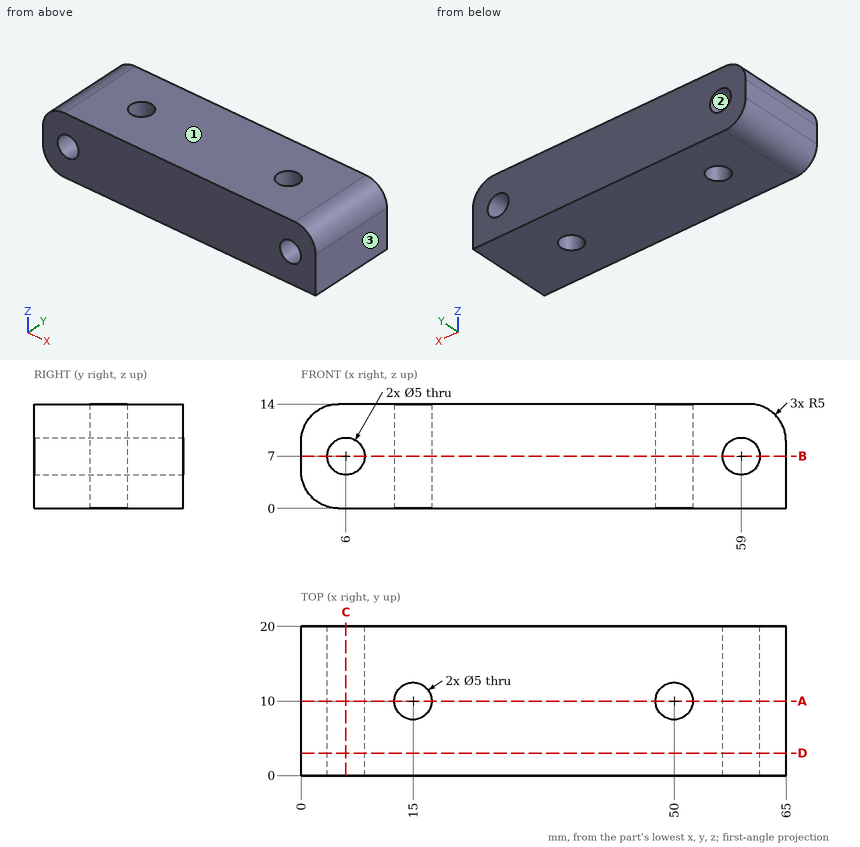
Input: dimensioned drawing with shaded views. Units: mm. Origin: part minimum x, y, z. Round coordinates to 2 decimals unless told otherwise and drop trailing zeros. Order: outer loops, then holes, each group sorted by start corner. A loop starts at its lowest first (then second) coordinate and runs counter-clockwise, first axis right, second up. Notation, with made-up numbers: (-2.75, 45) - (45.25, 45) arc R24 ccw to (45.25, 79) - close; hole circle Ø2 at (56, -39). An arc over 180 degrees is marked (long way). Answer as a JSON object with one key per item and string values. Group by question number.
(1) Cut plane C-C (x = 6). Return loops of the section in (y, z).
(2) Cut plane A-A (y = 10). Return loops of the section in (x, z).
(3) Pin query (flat end, axial travel): P1, Ø2, axis at y = 3, z = 2.5, coming from the -X side; P2, Ø1, axis at y = 3.5, z = 1.5, coming from the -X side. Return the tip coordinate at first contact, or that it passes through.
(4) Cut plane D-D (y = 3). Return loops of the section in (x, z), then the cut area to 3 significant figures.
(5) Cut plane B-B (z = 7). Return loops of the section in (x, y).
(6) Material intervals for probe 1 along Z at (x, y) = (59, 4); probe 2 along Y at (x, z) = (50, 8); probe 3 along X at (y, z) = (6.75, 5.25), sorted ascending. Write a range as from..to.
(7) Draft query along X for the marked faces 1, 2 and 3. Return one class per face: released by +X, released by -X, zero draft, split by the parting line, or undercut.
Here are the results:
{
 "1": {"outline": "(0, 0) - (20, 0) - (20, 4.5) - (0, 4.5) - close; (0, 9.5) - (20, 9.5) - (20, 14) - (0, 14) - close"},
 "2": {"outline": "(0, 5) arc R5 ccw to (5, 0) - (12.5, 0) - (12.5, 14) - (5, 14) arc R5 ccw to (0, 9) - close; (17.5, 0) - (47.5, 0) - (47.5, 14) - (17.5, 14) - close; (52.5, 0) - (65, 0) - (65, 9) arc R5 ccw to (60, 14) - (52.5, 14) - close; hole circle Ø5 at (6, 7); hole circle Ø5 at (59, 7)"},
 "3": {"P1": "stops at x = 0.23", "P2": "stops at x = 1"},
 "4": {"outline": "(0, 5) arc R5 ccw to (5, 0) - (65, 0) - (65, 9) arc R5 ccw to (60, 14) - (5, 14) arc R5 ccw to (0, 9) - close; hole circle Ø5 at (6, 7); hole circle Ø5 at (59, 7)", "area": "855 mm^2"},
 "5": {"outline": "(0, 0) - (3.5, 0) - (3.5, 20) - (0, 20) - close; (8.5, 0) - (56.5, 0) - (56.5, 20) - (8.5, 20) - close; (61.5, 0) - (65, 0) - (65, 20) - (61.5, 20) - close; hole circle Ø5 at (15, 10); hole circle Ø5 at (50, 10)"},
 "6": {"probe 1": "z = 0..4.5, 9.5..14", "probe 2": "y = 0..7.5, 12.5..20", "probe 3": "x = 0..4.21, 7.79..57.21, 60.79..65"},
 "7": {"face 1": "zero draft", "face 2": "undercut", "face 3": "released by +X"}
}
